```python
from build123d import *

# Parameters (mm, degrees)
F0_W     = 91.748398
F0_H     = 91.2087
F1_DEPTH = 25.4
F4_D     = 50.8
F2_R     = 25.893128
F6_DEPTH = 63.246
F7_D     = 38.1


with BuildPart() as f1:
    # F0 (on Front) → F1 (new body)
    with BuildSketch(Plane.XZ):
        with Locations((2.158785, -0.944471)):
            Rectangle(F0_W, F0_H)
    extrude(amount=F1_DEPTH)

    # F4 (through all)
    with Locations(Plane.XZ.offset(25.4)):
        with Locations((0, 0)):
            Hole(F4_D / 2)

    # F2 (on face) → F6 (join)
    with BuildSketch(Plane.XZ.offset(25.4)):
        Circle(F2_R)
    extrude(amount=-F6_DEPTH)

    # F7 (through all)
    with Locations(Plane.XZ.offset(25.4)):
        with Locations((0, 0)):
            Hole(F7_D / 2)


solid = f1.part
```
Geometry check sheet. Reference: the model listing, model coordinates, mm. A direction names the side the tool comes from. Give positions to 0.01 mm unless a question says otherwise; leave off trailing zeros. Order: outer loops, then holes, each group sorted by start corner. A loop starts at its lowest first (then second) coordinate and runs counter-clockwise, first axis right, second up. Notation, with made-up numbers: (4, 34) -> (13, 34) arc R27 ccw to (13, 54) -> close; hole circle Ø10 at (-19.75, -36.75). An arc over 180 degrees is marked (long way). Write each question's results on one line, items separated by ' | '. Start each with the question number.
(1) Scan lines: line 1 (Z direction, x = 0, y = -2); line 2 (Z direction, x = 0, y = 22); line 3 (Y direction, x = 31, z = 3.5). Record each from-to range of solid material in increasing order.
(2) Gauge pin test, flat ends, axial feed: P1, Ø1, axis at y = 4.5, z = -11.5, coming from the +X side; P2, Ø6, axis at x = -21.5, y = 27, coming from the +Z side; P3, Ø8, axis at y = 7, z = -25.5, coming from the -X side. Record the tip position at first contact, or that the pin passes through.
(3) Access from +Z, -Z, +X, -X, +Y, -Y to the whole of each face (thin tool, end or side, straight path). Record for faces 4 (the face through (-3.371, 18.658, 25.673)), 5 (the face through (2, -13, 44.66)).
(4) Sectioned sample at C-C (y = 22). Enter the section's corners in (x, z), plus the area to 3 significant figures.
(5) Sectioned sample at D-D (z = 28). Enter the section's corners in (x, y), plus the area to 3 significant figures.
(6) Sectioned sample at B-B (x = -5.5). Enter the section's corners in (y, z).
(7) Mould release check, pull along X, two halves, no side actions. Record for faces 1 (the face through (-14, 37.846, 14)), 2 (the face through (15.12, 6.67, -11.59)), 3 (the face through (48.033, -13, -2)): pulls with the +X half, pulls with the -X half, needs draft (parallel to the pull), parting line crosses it, or undercut.
(8) Sectioned sample at A-A (z = 0). Enter the section's corners in (x, y).
Answer below:
1) line 1: -46.55 to -19.05, 19.05 to 44.66 | line 2: -25.89 to -19.05, 19.05 to 25.89 | line 3: -25.4 to 0
2) P1: x = 23.44 | P2: z = 18.12 | P3: x = -14.43
3) face 4: +Y | face 5: +Z, +X, -X, +Y, -Y
4) outline: circle Ø51.79 at (0, 0); hole circle Ø38.1 at (0, 0) | area: 966 mm2
5) outline: (-43.72, -25.4) -> (48.03, -25.4) -> (48.03, 0) -> (-43.72, 0) -> close | area: 2,330 mm2
6) outline: (-25.4, -46.55) -> (0, -46.55) -> (0, -25.3) -> (37.85, -25.3) -> (37.85, -18.24) -> (-25.4, -18.24) -> close; (-25.4, 18.24) -> (37.85, 18.24) -> (37.85, 25.3) -> (0, 25.3) -> (0, 44.66) -> (-25.4, 44.66) -> close
7) face 1: needs draft | face 2: undercut | face 3: pulls with the +X half
8) outline: (-43.72, -25.4) -> (-19.05, -25.4) -> (-19.05, 37.85) -> (-25.89, 37.85) -> (-25.89, 0) -> (-43.72, 0) -> close; (19.05, -25.4) -> (48.03, -25.4) -> (48.03, 0) -> (25.89, 0) -> (25.89, 37.85) -> (19.05, 37.85) -> close
